Autodesk Inventor part; units mm, degrees
ref_plane "Work Plane1" through (0, 57, 120) normal (0, 1, 0) x (-1, 0, 0)
ref_plane "YZ Plane" through (0, 0, 0) normal (1, 0, 0) x (0, 1, 0)
ref_plane "XZ Plane" through (0, 0, 0) normal (0, 1, 0) x (-1, 0, 0)
sketch "Sketch1" plane through (0, 0, 0) normal (0, 0, 1) x (1, 0, 0)
  circle A0 centre (0, 0) radius 57
  circle A1 centre (0, 0) radius 55
  dimension "d0" = 114
  dimension "d1" = 110
extrude "Extrusion1" add sketch "Sketch1" along normal blind 120
sketch "Sketch2" plane through (0, 0, 120) normal (0, 0, 1) x (1, 0, 0)
  circle A0 centre (0, 0) radius 57
  point P0 (0, 57)
ref_plane "Work Plane1" through (0, 57, 120) normal (0, 1, 0) x (-1, 0, 0)
sketch "Sketch3" plane through (0, 57, 120) normal (0, 1, 0) x (-1, 0, 0)
  line L0 (57, 0) -> (-57, 0)
  point P0 (0, -120)
  point P1 (0, -50)
  dimension "d4" = 50
hole "Hole1" at (0, 57, 70) direction (0, -1, 0) diameter 10 depth 20 tip angle 118
sketch "Sketch6" plane through (0, 0, 120) normal (0, 0, 1) x (1, 0, 0)
  circle A0 centre (0, 0) radius 57
  point P0 (0, 57)
sketch "Sketch11" plane through (0, 0, 120) normal (0, 0, 1) x (1, 0, 0)
  circle A0 centre (0, 0) radius 57
  line L0 (28.5, 49.3634) -> (0, 0)
  line L1 (57, 0) -> (0, 0)
  dimension "d47" = 60
ref_plane "Work Plane7" through (28.5, 49.3634, 120) normal (0.5, 0.8660254, 0) x (-0.8660254, 0.5, 0)
sketch "Sketch12" plane through (28.5, 49.3634, 120) normal (0.5, 0.8660254, 0) x (-0.8660254, 0.5, 0)
  line L0 (57, 0) -> (-57, 0)
  point P0 (0, -120)
  point P1 (0, -17.607)
  dimension "d48" = 17.607
hole "Hole6" at (28.5, 49.3634, 102.393) direction (-0.5, -0.8660254, 0) diameter 2 end through all
equation "\"d54\" = Thickness"
equation "\"BendRadius\" = Thickness"
equation "\"BendReliefWidth\" = Thickness"
equation "\"BendReliefDepth\" = 0.5 * Thickness"
equation "\"CornerReliefSize\" = 4 * Thickness"
equation "\"MinimumRemnant\" = 2 * Thickness"
equation "\"TransitionRadius\" = BendRadius"
equation "\"JacobiRadiusSize\" = BendRadius"
equation "\"GapSize\" = Thickness"
properties part number "Electromagnetic cover body"
Input: part model. Units: mm. Frame: model coordinates. Coordinates: 2 decimals unless noted, no trailing zeros. Write each loop counter-clockwise with the first axis right and the second up, starting at its lowest first coordinate (ties: lowest second). Pieces come first, ordered by that corner, then holes. Notation, with made-up numbers: M 50,35 L 75,35 A19 cw 75,63 Z; hole C -10,40.5 d9. An arc over 180 degrees is marked long. Answer as a JSON object with one key per item and string values. Group by question number.
(1) Section C-C on x = -41. Output: boundary loops of the cut face in (y, z).
(2) Ray query, line 1 along X through (y, z) = (-2, 58.5); line 2 along Y through (x, z) = (0, 48.5); line 3 along Z through (x, y) = (0, 55.9). Return the intervals inside material, ascending. Write a range as [from, to].
(3) Mould query, pull axis Z, two halves, no side actions, for faces 1 (the face through (0, 56, 65)), 2 (the face through (-30, 47, 0)), 3 (the face through (-30, 47, 120)). Classes: pulls with the +Z half, pulls with the -Z half, needs draft (parallel to the pull), parting line crosses it, or undercut.
(4) Section A-A on x = 0. Output: boundary loops of the cut face in (y, z).
(5) Section D-D on z = 38. Output: boundary loops of the cut face in (x, y).
(6) Contact query for flat-ended pins moving along their axis: P1, Ø8, axis at y = 15.5, z = 84, coming from the -X side; P2, Ø2, axis at y = 24.5, z = 29, coming from the +X side; P3, Ø16, axis at x = 0, z = 70, coming from the -Y side. Output: stop coordinate, or through.
(7) Section B-B on y = 0. Output: boundary loops of the cut face in (x, z).
Result set:
{
 "1": {"outline": "M -39.6,0 L -36.66,0 L -36.66,120 L -39.6,120 Z; M 36.66,0 L 39.6,0 L 39.6,120 L 36.66,120 Z"},
 "2": {"line 1": "x = [-56.96, -54.96], [54.96, 56.96]", "line 2": "y = [-57, -55], [55, 57]", "line 3": "z = [0, 65], [75, 120]"},
 "3": {"face 1": "undercut", "face 2": "pulls with the -Z half", "face 3": "pulls with the +Z half"},
 "4": {"outline": "M -57,0 L -55,0 L -55,120 L -57,120 Z; M 55,0 L 57,0 L 57,65 L 55,65 Z; M 55,75 L 57,75 L 57,120 L 55,120 Z"},
 "5": {"outline": "C 0,0 d114; hole C 0,0 d110"},
 "6": {"P1": "stops at x = -55.83", "P2": "stops at x = 51.93", "P3": "stops at y = -57"},
 "7": {"outline": "M -57,0 L -55,0 L -55,120 L -57,120 Z; M 55,0 L 57,0 L 57,120 L 55,120 Z"}
}
